Design review of the part built by this model. Coordinates are the model's own, in mm. A direction names the side the tool comes from. Coordinates: 2 decimals unless noted, no trailing zeros. Order: outer loops, then holes, each group sorted by start corner. A loop starts at its lowest first (then second) coordinate and runs counter-clockwise, first axis right, second up. Notation, with made-up numbers: (-8.75, -6.5) - (35.25, -6.5) arc R27 ccw to (35.25, 25.5) - close; hole circle Ø7 at (27.5, 87). An arc over 180 degrees is marked (long way). Write each question's results on one line, items separated by ' | '. Start each with the question number.
```python
from build123d import *

# Parameters (mm, degrees)
SKETCH_1_W      = 92.5
SKETCH_1_H      = 92.5
SKETCH_1_R      = 2
EXTRUDE_1_DEPTH = 25.4
FILLET_2_R      = 3


with BuildPart() as part:
    # Эскиз1 → Бобышка-Вытянуть1 (new body)
    with BuildSketch(Plane.XY):
        Rectangle(SKETCH_1_W, SKETCH_1_H)
        with Locations((-41.35, 41.35)):
            Circle(SKETCH_1_R, mode=Mode.SUBTRACT)
        with Locations((-41.35, -41.35)):
            Circle(SKETCH_1_R, mode=Mode.SUBTRACT)
        with Locations((41.35, -41.35)):
            Circle(SKETCH_1_R, mode=Mode.SUBTRACT)
        with Locations((41.35, 41.35)):
            Circle(SKETCH_1_R, mode=Mode.SUBTRACT)
        with BuildLine():
            Line((30.103737124, 25.18585935), (10.244232434, 18.036233028))
            ThreePointArc((10.244232434, 18.036233028), (8.93715954, 16.402747815), (9.801515353, 14.497596242))
            ThreePointArc((9.801515353, 14.497596242), (13.81482208, 10.742471359), (16.465475636, 5.92774089))
            Line((16.465475636, 5.92774089), (28.365935027, -27.128144611))
            ThreePointArc((28.365935027, -27.128144611), (39.228362099, -1.303114362), (30.103737124, 25.18585935))
        make_face(mode=Mode.SUBTRACT)
        with BuildLine():
            Line((5.92774089, -16.465475636), (-27.128144611, -28.365935027))
            ThreePointArc((-27.128144611, -28.365935027), (-1.303114362, -39.228362099), (25.18585935, -30.103737124))
            Line((25.18585935, -30.103737124), (18.036233028, -10.244232434))
            ThreePointArc((18.036233028, -10.244232434), (16.402747815, -8.93715954), (14.497596242, -9.801515353))
            ThreePointArc((14.497596242, -9.801515353), (10.742471359, -13.81482208), (5.92774089, -16.465475636))
        make_face(mode=Mode.SUBTRACT)
        with BuildLine():
            Line((-16.465475636, -5.92774089), (-28.365935027, 27.128144611))
            ThreePointArc((-28.365935027, 27.128144611), (-39.228362099, 1.303114362), (-30.103737124, -25.18585935))
            Line((-30.103737124, -25.18585935), (-10.244232434, -18.036233028))
            ThreePointArc((-10.244232434, -18.036233028), (-8.93715954, -16.402747815), (-9.801515353, -14.497596242))
            ThreePointArc((-9.801515353, -14.497596242), (-13.81482208, -10.742471359), (-16.465475636, -5.92774089))
        make_face(mode=Mode.SUBTRACT)
        with BuildLine():
            Line((-5.92774089, 16.465475636), (27.128144611, 28.365935027))
            ThreePointArc((27.128144611, 28.365935027), (1.303114362, 39.228362099), (-25.18585935, 30.103737124))
            Line((-25.18585935, 30.103737124), (-18.036233028, 10.244232434))
            ThreePointArc((-18.036233028, 10.244232434), (-16.402747815, 8.93715954), (-14.497596242, 9.801515353))
            ThreePointArc((-14.497596242, 9.801515353), (-10.742471359, 13.81482208), (-5.92774089, 16.465475636))
        make_face(mode=Mode.SUBTRACT)
    extrude(amount=EXTRUDE_1_DEPTH)

    # Скругление2
    fillet_2_edges = [part.edges().sort_by_distance(p)[0] for p in [
        (-46.25, 46.25, 12.7),
        (46.25, 46.25, 12.7),
        (46.25, -46.25, 12.7),
        (-46.25, -46.25, 12.7),
    ]]
    fillet(fillet_2_edges, radius=FILLET_2_R)


solid = part.part
```
(1) Take a section at C-C (z = 18). State how many separate pieces and enclosed holes the cut face has, plus the area to 3 significant figures.
(2) Take a section at A-A (y = 41.35). State the section outline as (x, z) points, plus the area to 3 significant figures.
(3) Take a section at D-D (y = -23). State the section outline as (x, z) points.
(4) To check wall thickness, follow line 1 along Y through (x, z) = (-41.35, 16.5); line 2 along X through (y, z) = (5, 11.25); line 3 along X through (y, z) = (-6.5, 9.25). State the ranges of each line that lie inside material, in increasing order. Write a range as [from, to].
(5) Mouldability with a two-part tool opening along Y and no side actions: class faces 1 (the face through (42.273, 39.576, 12.522)), 2 (the face through (46.25, -1, 13)), 3 (the face through (45.35, -45.39, 12.88)) as +Y half, -Y half, draft (parallel to the pull), parting line (faces both ways), or undercut.
(6) Tool access review of faces 4 (the face through (10.369, 22.332, 12.522)), 5 (the face through (-1, 1, 0)): name each direction out of +Z, -Z, +X, -X, +Y, -Y from which nothing blocks a thin tool from reaching the whole face with its end or side.
Worked out:
1) separate pieces: 1 | enclosed holes: 8 | area: 5,090 mm^2
2) outline: (-46.25, 0) - (-43.35, 0) - (-43.35, 25.4) - (-46.25, 25.4) - close; (-39.35, 0) - (39.35, 0) - (39.35, 25.4) - (-39.35, 25.4) - close; (43.35, 0) - (46.25, 0) - (46.25, 25.4) - (43.35, 25.4) - close | area: 2,150 mm^2
3) outline: (-46.25, 0) - (-31.81, 0) - (-31.81, 25.4) - (-46.25, 25.4) - close; (-24.03, 0) - (-12.22, 0) - (-12.22, 25.4) - (-24.03, 25.4) - close; (22.63, 0) - (26.88, 0) - (26.88, 25.4) - (22.63, 25.4) - close; (31.81, 0) - (46.25, 0) - (46.25, 25.4) - (31.81, 25.4) - close
4) line 1: [-46.25, -43.35], [-39.35, 39.35], [43.35, 46.25] | line 2: [-46.25, -38.93], [-20.4, 16.8], [38.93, 46.25] | line 3: [-46.25, -38.71], [-16.25, 20.94], [38.71, 46.25]
5) face 1: undercut | face 2: draft | face 3: -Y half
6) face 4: +Z, -Z | face 5: -Z, +X, -X, +Y, -Y
